from build123d import *

# Parameters (mm, degrees)
EXTRUSION1_DEPTH = 19
ESQUISSE2_R      = 1.5
EXTRUSION2_DEPTH = 5
ESQUISSE3_R      = 2
EXTRUSION3_DEPTH = 47.241826523


with BuildPart() as part:
    # Esquisse1 → Extrusion1 (new body)
    with BuildSketch(Plane.XY):
        Polygon((18.706066256, -17.112080516), (18.706066256, -37.112080516), (38.706066256, -37.112080516), (38.706066256, -17.112080516), (37.206066256, -17.112080516), (37.206066256, -35.612080516), (20.206066256, -35.612080516), (20.206066256, -17.112080516), align=None)
    extrude(amount=EXTRUSION1_DEPTH)

    # Esquisse2 → Extrusion2 (cut)
    with BuildSketch(Plane.XZ.offset(37.112080516)):
        with Locations(Location((23.706066256, 9.5, 0), (0, 0, 270))):
            Circle(ESQUISSE2_R)
        with Locations(Location((33.706066256, 9.5, 0), (0, 0, 270))):
            Circle(ESQUISSE2_R)
    extrude(amount=-EXTRUSION2_DEPTH, mode=Mode.SUBTRACT)

    # Esquisse3 → Extrusion3 (cut, through all)
    with BuildSketch(Plane.ZY.offset(-18.706066256)):
        with Locations(Location((9.5, -25.112080516, 0), (0, 0, 270))):
            Circle(ESQUISSE3_R)
    extrude(amount=-EXTRUSION3_DEPTH, mode=Mode.SUBTRACT)


solid = part.part
Geometry: final body of the model. Coordinates: model frame, mm. A direction names the side the tool comes from. Round coordinates to 2 decimals unless told otherwise and drop trailing zeros. Loops run counter-clockwise (first coordinate to the right, second up) from the corner with the lowest first, then second, coordinate; pieces in that order, holes last.
Q1. Pin query (flat end, axial travel): P1, Ø2.5, axis at y = -25.11, z = 9.5, coming from the -X side; P2, Ø5, axis at x = 31.5, z = 5, coming from the +Y side. Return the tip coordinate at first contact, or that it passes through.
Q2. Section B-B on z = 9.5. Return loops of the section in (x, y), plus the area to 3 significant figures.
Q3. Material intervals for L1, parallel to X at y = -36.3, z = 9.5; L2, parallel to X at y = -33.5, z = 18.25; L3, parallel to Y at x = 34.5, z = 5, sorted ascending.
Q4. Section C-C on x = 23.25. Return loops of the section in (y, z), plus the area to 3 significant figures.
Q5. Pull-direction query (X, two-part tool) for faces 3 (the flat face through (29, -37.112, 9)), 4 (the flat face through (18.706, -27, 7)), 5 (the flat face through (29, -35.612, 9)), 6 (the flat face through (20.206, -29, 9)); classes: released by +X, released by -X, zero draft, split by the parting line, or undercut.
Q6. Section D-D on z = 3.75. Return loops of the section in (x, y), plus the area to 3 significant figures.
Q7. Section A-A on y = -33.75. Return loops of the section in (x, z), plus the area to 3 significant figures.
Q8. Access query for faces 1 (the flat face through (37.206, -28, 9)), 2 (the cylindrical face through (35.193, -36.373, 9.695)). Directions: +Z, -Z, +X, -X, +Y, -Y. A direction counts if a zero-diameter tool reaches every point of the face in a straight line with its end or side. Return the directions, or none.
Evaluation:
1. P1: passes through
1. P2: stops at y = -35.61
2. outline: (18.71, -37.11) - (22.21, -37.11) - (22.21, -35.61) - (20.21, -35.61) - (20.21, -27.11) - (18.71, -27.11) - close; (18.71, -23.11) - (20.21, -23.11) - (20.21, -17.11) - (18.71, -17.11) - close; (25.21, -37.11) - (32.21, -37.11) - (32.21, -35.61) - (25.21, -35.61) - close; (35.21, -37.11) - (38.71, -37.11) - (38.71, -27.11) - (37.21, -27.11) - (37.21, -35.61) - (35.21, -35.61) - close; (37.21, -23.11) - (38.71, -23.11) - (38.71, -17.11) - (37.21, -17.11) - close
2. area: 64.5 mm2
3. L1: x = 18.71 to 22.21, 25.21 to 32.21, 35.21 to 38.71
3. L2: x = 18.71 to 20.21, 37.21 to 38.71
3. L3: y = -37.11 to -35.61
4. outline: (-37.11, 0) - (-35.61, 0) - (-35.61, 8.07) - (-37.11, 8.07) - close; (-37.11, 10.93) - (-35.61, 10.93) - (-35.61, 19) - (-37.11, 19) - close
4. area: 24.2 mm2
5. face 3: zero draft
5. face 4: released by -X
5. face 5: undercut
5. face 6: undercut
6. outline: (18.71, -37.11) - (38.71, -37.11) - (38.71, -17.11) - (37.21, -17.11) - (37.21, -35.61) - (20.21, -35.61) - (20.21, -17.11) - (18.71, -17.11) - close
6. area: 85.5 mm2
7. outline: (18.71, 0) - (20.21, 0) - (20.21, 19) - (18.71, 19) - close; (37.21, 0) - (38.71, 0) - (38.71, 19) - (37.21, 19) - close
7. area: 57.0 mm2
8. face 1: +Z, -Z, +Y
8. face 2: +Y, -Y
